Input: dimensioned drawing with shaded views. Units: mm. Origin: part minimum x, y, z. A direction names the side the tool comes from. Coordinates: 2 decimals unless noted, no trailing zeros. Loops run counter-clockwise (first coordinate to the right, second up) from the corner with the lowest first, then second, coordinate; pieces in that order, holes last.
Item 1: Section D-D on y = 22. Return loops of the section in (x, z).
Item 2: Section C-C on x = 46. Return loops of the section in (y, z), and give its area (3 significant figures).
Item 3: Reachability of the marked faces 1 and 2 from +Z, -Z, +X, -X, +Y, -Y: full face, straight path, thin tool, end or side. Return the list, or none.
Item 4: Ray query, line 1 along X through (y, z) = (14.25, 4.75); line 2 along Y through (x, z) = (46, 4.85); line 3 along X through (y, z) = (27.25, 2.8). Return the intervals inside material, ascending.
Item 5: Contact query for a flat-ended pin moving along its axis: P1, Ø1.5, axis at y = 14.5, z = 3, coming from the -X side. Output: stop coordinate, or through.
Item 6: Section A-A on y = 8.75. Return loops of the section in (x, z), and give its area (3 significant figures).
Item 7: Pull-direction query (X, two-part tool) for the marked faces 3, 4 and 5; classes: released by +X, released by -X, zero draft, split by the parting line, or undercut.
Item 8: Section B-B on z = 2.85. Return loops of the section in (x, y).
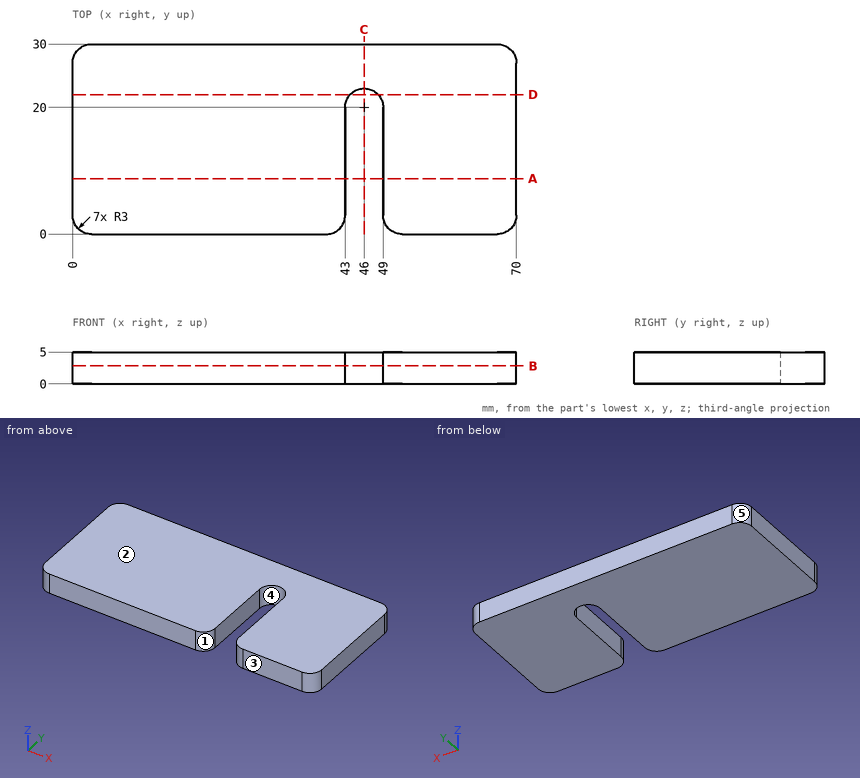
Results found:
1. outline: (0, 0) - (43.76, 0) - (43.76, 5) - (0, 5) - close; (48.24, 0) - (70, 0) - (70, 5) - (48.24, 5) - close
2. outline: (23, 0) - (30, 0) - (30, 5) - (23, 5) - close
2. area: 35.0 mm2
3. face 1: +Z, -Z, -Y
3. face 2: +Z, +X, -X, +Y, -Y
4. line 1: x = 0 to 43, 49 to 70
4. line 2: y = 23 to 30
4. line 3: x = 0.01 to 69.99
5. P1: stops at x = 0
6. outline: (0, 0) - (43, 0) - (43, 5) - (0, 5) - close; (49, 0) - (70, 0) - (70, 5) - (49, 5) - close
6. area: 320 mm2
7. face 3: zero draft
7. face 4: undercut
7. face 5: released by -X
8. outline: (0, 3) arc R3 ccw to (3, 0) - (40, 0) arc R3 ccw to (43, 3) - (43, 20) arc R3 cw to (49, 20) - (49, 3) arc R3 ccw to (52, 0) - (67, 0) arc R3 ccw to (70, 3) - (70, 27) arc R3 ccw to (67, 30) - (3, 30) arc R3 ccw to (0, 27) - close
